Can you work these out from the model? Positions are in its coordinate system, mm. Face numbers are marked on the shaded views. A direction names the side the tool comes from. Round coordinates to 2 decimals unless told otherwise and drop trailing zeros. Order: outer loops, then holes, each group sorted by start corner. A loop starts at its lowest first (then second) coordinate and runs counter-clockwise, first axis right, second up.
Q1. If I drill on line 1 (Y direction, x = 0, z = 13); line 2 (X direction, y = 1.25, z = 3.5); line 3 (X direction, y = 2.5, z = 0), over which ranges is the centre line in solid material (lowest first)?
Q2. If we section it at B-B (z = 0): Please give me the cut outline in (x, y).
Q3. We'd pull the mould along X, two halves only. Please class the marked faces 1 and 2: pulls with the +X half, pulls with the -X half, needs draft (parallel to the pull), parting line crosses it, or undercut.
Q4. If we section it at C-C (x = 60): Please give me the cut outline in (y, z).
Q5. For the marked faces 3, 4 and 5, which set-ups out of +Z, -Z, +X, -X, +Y, -Y let a thin tool reach every point of the face, with its end or its side?
Q6. If we section it at D-D (x = -32.5): Please give me the cut outline in (y, z), plus the area to 3 significant figures.
Q7. If we section it at A-A (x = 0): Please give me the cut outline in (y, z), plus the area to 3 significant figures.
Q8. Will these pins go through, and if not, where does the flat tip stop? P1, Ø4, axis at y = 0, z = -2.5, coming from the -X side; P2, Ø6, axis at x = 49.5, y = -2, coming from the +Z side; P3, Ø6, axis at x = -8.5, z = -14, coming from the +Y side.
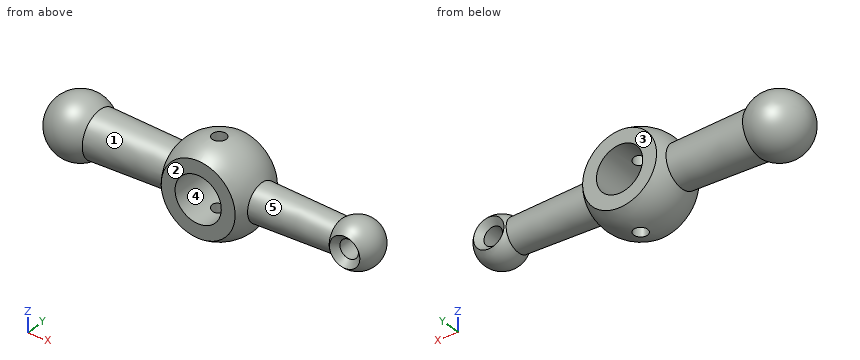
from build123d import *

# Parameters (mm, degrees)
CHAMFER_1_SIZE      = 3
SKETCH_3_R          = 3
CUT_EXTRUDE_1_DEPTH = 50


with BuildPart() as part:
    # Эскиз1 → Повернуть1 (revolve)
    with BuildSketch(Plane.XY):
        with BuildLine():
            Line((-51.693376137, 10), (-17.843804593, 9.033196425))
            ThreePointArc((-17.843804593, 9.033196425), (0.571002482, 19.991847242), (18.33030278, 8))
            Line((18.33030278, 8), (52.871765135, 7.013434801))
            ThreePointArc((52.871765135, 7.013434801), (63.789304115, 9.254251689), (70, 0))
            Line((70, 0), (-73, 0))
            ThreePointArc((-73, 0), (-65.523309234, 11.768307232), (-51.693376137, 10))
        make_face()
    revolve(axis=Axis((-73, 0, 0), (1, 0, 0)))

    # Эскиз2 → Вырез-Повернуть1 (revolve, cut)
    with BuildSketch(Plane.XY, mode=Mode.PRIVATE) as cut_revolve_1_sk:
        with BuildLine():
            Line((0, -12), (0, 12))
            Line((0, 12), (0, 20))
            ThreePointArc((0, 20), (8.94427191, 17.88854382), (16, 12))
            Line((16, 12), (10, 12))
            Line((10, 12), (10, -12))
            Line((10, -12), (16, -12))
            ThreePointArc((16, -12), (8.94427191, -17.88854382), (0, -20))
            Line((0, -20), (0, -12))
        make_face()
    revolve(cut_revolve_1_sk.sketch.rotate(Axis((0, 0, 0), (0, 1, 0)), 90), axis=Axis((0, 0, 0), (0, 1, 0)), mode=Mode.SUBTRACT)

    # Эскиз2<3> → Вырез-Повернуть2 (revolve, cut)
    with BuildSketch(Plane.XY):
        Polygon((66, -8), (66, -15.272316645), (60, -15.272316645), (60, 15.272316645), (66, 15.272316645), (66, 8), (64, 8), (64, -8), align=None)
    revolve(axis=Axis((60, -15.272316645, 0), (0, 1, 0)), mode=Mode.SUBTRACT)

    # Фаска1
    # the kernel refuses this chamfer: 3 mm, written as the material it takes off along each edge
    with BuildSketch(Plane(origin=(60, -8, 0), x_dir=(1, 0, 0), z_dir=(0, 0, 1))) as chamfer_1_piece_1:
        Polygon((4 + CHAMFER_1_SIZE, 0), (4, CHAMFER_1_SIZE), (4, 0), align=None)
    revolve(axis=Axis((60, -8, 0), (0, 1, 0)), mode=Mode.SUBTRACT)
    with BuildSketch(Plane(origin=(60, 8, 0), x_dir=(1, 0, 0), z_dir=(0, 0, 1))) as chamfer_1_piece_2:
        Polygon((4 + CHAMFER_1_SIZE, 0), (4, -CHAMFER_1_SIZE), (4, 0), align=None)
    revolve(axis=Axis((60, 8, 0), (0, 1, 0)), mode=Mode.SUBTRACT)

    # Эскиз3 → Вырез-Вытянуть1 (cut, symmetric)
    with BuildSketch(Plane.XY):
        Circle(SKETCH_3_R)
    extrude(amount=CUT_EXTRUDE_1_DEPTH, both=True, mode=Mode.SUBTRACT)


solid = part.part
Solution:
1. line 1: y = -12 to -3, 3 to 12
1. line 2: x = -72.46 to -9.37, 9.37 to 58.06, 61.94 to 69.28
1. line 3: x = -72.76 to -10, 10 to 56, 64 to 69.68
2. outline: (-51.69, -10) - (-17.84, -9.03) arc R20 ccw to (-16, -12) - (-10, -12) - (-10, 12) - (-16, 12) arc R20 ccw to (-17.84, 9.03) - (-51.69, 10) arc R13 ccw (long way) to start; (10, -12) - (16, -12) arc R20 ccw to (18.33, -8) - (52.87, -7.01) arc R10 ccw to (53.45, -7.55) - (56, -5) - (56, 5) - (53.45, 7.55) arc R10 ccw to (52.87, 7.01) - (18.33, 8) arc R20 ccw to (16, 12) - (10, 12) - close; (64, -5) - (66.55, -7.55) arc R10 ccw to (66.55, 7.55) - (64, 5) - close
3. face 1: undercut
3. face 2: needs draft
4. outline: (-7.55, -6.55) arc R10 ccw to (7.55, -6.55) - (5, -4) - (-5, -4) - close; (-7.55, 6.55) - (-5, 4) - (5, 4) - (7.55, 6.55) arc R10 ccw to start
5. face 3: +Z, -Z, +X, +Y
5. face 4: +Y, -Y
5. face 5: none
6. outline: circle Ø18.9 at (0, 0)
6. area: 281 mm2
7. outline: (-12, -16) arc R20 ccw to (-3, -19.77) - (-3, -10) - (-12, -10) - close; (-12, 10) - (-3, 10) - (-3, 19.77) arc R20 ccw to (-12, 16) - close; (3, -19.77) arc R20 ccw to (12, -16) - (12, -10) - (3, -10) - close; (3, 10) - (12, 10) - (12, 16) arc R20 ccw to (3, 19.77) - close
7. area: 300 mm2
8. P1: stops at x = -72.99
8. P2: stops at z = 7.18
8. P3: stops at y = 12
